Can you work these out from the model? Positions are in its coordinate system, mm. A direction names the side the tool comes from. Round coordinates to 2 decimals unless told otherwise and drop trailing zeros. Write each loop counter-clockwise with the first axis right and the second up, starting at its lowest first coordinate (ties: lowest second). Pieces come first, ordered by that corner, then holes. Notation, with made-up numbers: M 33.5,83 L 80.5,83 A22 cw 80.5,122 Z; hole C 66.25,29 d1. An arc over 180 degrees is marked long. Answer in a Markdown table with one row per item. Add a question column.
(1) I'm going to push flat-ended pins straight in: pin 1 (2.5 mm diameter, centred on x = 29.28, z = 1.31, fed in from -Y); pin 2 (2.5 mm diameter, centred on y = 1.5, z = 1.5, fed in from +X); pin 3 (3 mm diameter, centred on x = 16, z = -45.5, fed in from +Y). Where does each tip first touch, or does it pass through?
(2) Suppose I cut it at B-B, the plane x = 22.5. Write out the boundary of the cut face in (y, z).
(3) If I drill on probe 1 along Y at (x, z) = (34.5, -29.5); probe 2 along Z at (x, y) = (50.5, 0.7), over which ranges is the centre line in solid material (lowest first)?
(4) Suppose I cut it at C-C, the plane z = -10. Write out the boundary of the cut face in (x, y).
(5) For faces 4 (the face through (27.5, 2, -50)), 5 (the face through (31.5, 2, -50)), 6 (the face through (29, 3, 0)), 7 (the face through (14, 1, 0)), which set-ups out of +Z, -Z, +X, -X, +Y, -Y let a thin tool reach every point of the face, with its end or its side?
(6) Suppose I cut it at A-A, the plane y = 3.9. Write out the boundary of the cut face in (x, z), then the cut area to 3 significant figures.
(7) If we mould it in two halves opening along Z, with no side actions, what happens to faces 1 (the face through (29, 2, 3)), 2 (the face through (48, 1, -49)), 3 (the face through (29, 3, -49))? For each: released by +Z, released by -Z, zero draft, split by the parting line, or undercut.
from build123d import *

# Parameters (mm, degrees)
SKETCH1_W                                            = 64
SKETCH1_H                                            = 49
BOSS_EXTRUDE1_DEPTH                                  = 1.5
SKETCH4_W                                            = 4
SKETCH4_H                                            = 3
BOSS_EXTRUDE2_DEPTH                                  = 5
CSK_FOR_M1_6_COUNTERSUNK_FLAT_HEAD_SCREW_D           = 1.8
CSK_FOR_M1_6_COUNTERSUNK_FLAT_HEAD_SCREW_CSINK_D     = 3.6
CSK_FOR_M1_6_COUNTERSUNK_FLAT_HEAD_SCREW_CSINK_ANGLE = 90


with BuildPart() as part:
    # Sketch1 → Boss-Extrude1 (new body)
    with BuildSketch(Plane(origin=(0, 0, 0), x_dir=(1, 0, 0), z_dir=(0, 1, 0))):
        with Locations((32, 24.5)):
            Rectangle(SKETCH1_W, SKETCH1_H)
    extrude(amount=BOSS_EXTRUDE1_DEPTH)

    # Sketch4 → Boss-Extrude2 (add)
    with BuildSketch(Plane(origin=(0, 0, 0), x_dir=(1, 0, 0), z_dir=(0, 1, 0))):
        with Locations((29.5, -1.5)):
            Rectangle(SKETCH4_W, SKETCH4_H)
        with Locations((29.5, 50.5)):
            Rectangle(SKETCH4_W, SKETCH4_H)
    extrude(amount=BOSS_EXTRUDE2_DEPTH)

    # CSK for M1.6 Countersunk Flat Head Screw1 (through all)
    with Locations(Plane(origin=(0, 0, 0), x_dir=(-1, 0, 0), z_dir=(0, -1, 0))):
        with Locations((-29.279045155, 50.23733833), (-29.279045155, -1.306151962)):
            CounterSinkHole(CSK_FOR_M1_6_COUNTERSUNK_FLAT_HEAD_SCREW_D / 2, CSK_FOR_M1_6_COUNTERSUNK_FLAT_HEAD_SCREW_CSINK_D / 2, counter_sink_angle=CSK_FOR_M1_6_COUNTERSUNK_FLAT_HEAD_SCREW_CSINK_ANGLE)


solid = part.part
Calculated:
| question | item | result |
|---|---|---|
| 1 | pin 1 | y = 0.55 |
| 1 | pin 2 | x = 31.5 |
| 1 | pin 3 | y = 1.5 |
| 2 | outline | M 0,-49 L 1.5,-49 L 1.5,0 L 0,0 Z |
| 3 | probe 1 | 0 to 1.5 |
| 3 | probe 2 | -49 to 0 |
| 4 | outline | M 0,0 L 64,0 L 64,1.5 L 0,1.5 Z |
| 5 | face 4 | -Z, -X, +Y, -Y |
| 5 | face 5 | -Z, +X, +Y, -Y |
| 5 | face 6 | +X, -X, +Y |
| 5 | face 7 | +Z, -X, +Y, -Y |
| 6 | outline | M 27.5,-52 L 31.5,-52 L 31.5,-49 L 27.5,-49 Z; M 27.5,0 L 31.5,0 L 31.5,3 L 27.5,3 Z; hole C 29.28,-50.24 d1.8; hole C 29.28,1.31 d1.8 |
| 6 | area | 18.9 mm² |
| 7 | face 1 | released by +Z |
| 7 | face 2 | released by -Z |
| 7 | face 3 | undercut |
